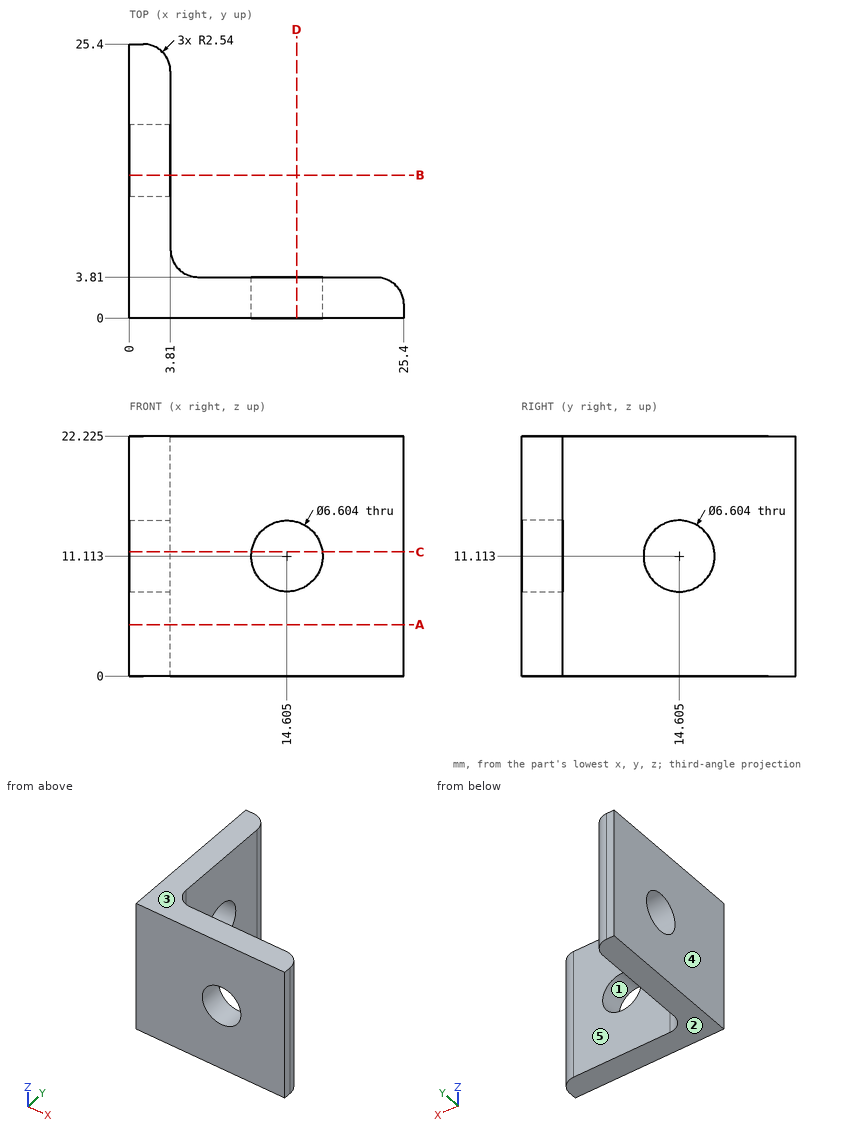
Answer from the drawing. Dimensions are ordinates in mm from the lowest x, y and z of the part. A direction names the side the tool comes from. Coordinates: 2 decimals unless noted, no trailing zeros. Write each loop counter-clockwise with the first axis right and the second up, starting at its lowest first coordinate (ties: lowest second). Pieces come first, ordered by that corner, then holes. Notation, with made-up numbers: M 44,39.25 L 67,39.25 A22 ccw 67,77.25 Z; hole C 0,62.25 d6. An arc over 180 degrees is marked long. Put each result on its own line as item: value. Start each with the question number.
1. A cutting plane is placed at D-D on x = 15.5. Write down the section's boundary in (y, z) (1 decimal).
2. Flat-ended cylindrical pins translate along their axes: P1, Ø4, axis at y = 10, z = 4.5, coming from the +X side; P2, Ø1, axis at x = 4, y = 8, coming from the -Z side; P3, Ø2, axis at x = 5.5, z = 8, coming from the +Y side; P4, Ø8, axis at x = 17, y = 8, coming from the +Z side. Find the tip coordinate at first contact, or state that the pin passes through.
3. A cutting plane is placed at A-A on z = 4.75. Write down the section's boundary in (x, y).
4. A cutting plane is placed at C-C on z = 11.5. Count the separate pieces of the cut face and the enclosed holes in it, then the cut area to 3 significant figures.
5. Which of the six approach directions +Z, -Z, +X, -X, +Y, -Y give full straight-line access (tool end or side, diameter ignored) to the marked faces 4 and 5?
6. A cutting plane is placed at B-B on y = 13.25. Write down the section's boundary in (x, z) (1 decimal).
7. Consider line 1 (X direction, y = 18.75, z = 11.5); line 2 (X direction, y = 5.5, z = 21) (1 decimal). Determine where each line is inside the solid, lowest interval first. Write a range as from..to.
8. For a pull along Z with two mould halves and no side action, classify the marked faces 1, 2 and 3 as pulls with the +Z half, pulls with the -Z half, needs draft (parallel to the pull), parting line crosses it, or undercut.
Resolved:
1. outline: M 0,0 L 3.8,0 L 3.8,7.9 L 0,7.9 Z; M 0,14.3 L 3.8,14.3 L 3.8,22.2 L 0,22.2 Z
2. P1: stops at x = 3.81
2. P2: stops at z = 0
2. P3: stops at y = 4.61
2. P4: passes through
3. outline: M 0,0 L 25.4,0 L 25.4,1.27 A2.54 ccw 22.86,3.81 L 6.35,3.81 A2.54 cw 3.81,6.35 L 3.81,22.86 A2.54 ccw 1.27,25.4 L 0,25.4 Z
4. separate pieces: 3
4. enclosed holes: 0
4. area: 128 mm2
5. face 4: +Z, -Z, -X, +Y, -Y
5. face 5: +Z, -Z, +X, +Y
6. outline: M 0,0 L 3.8,0 L 3.8,8.1 L 0,8.1 Z; M 0,14.1 L 3.8,14.1 L 3.8,22.2 L 0,22.2 Z
7. line 1: x = 0..3.81
7. line 2: x = 0..4
8. face 1: undercut
8. face 2: pulls with the -Z half
8. face 3: pulls with the +Z half
